For this review, take the finished solid that the model builds, in its own axes (mm). Face numbers are marked on the shaded views. A direction names the side the tool comes from. Round coordinates to 2 decimals unless told otherwise and drop trailing zeros. Write each loop counter-clockwise with the first axis right and the second up, starting at its lowest first coordinate (ties: lowest second). Pieces come first, ordered by that corner, then holes. Notation, with made-up numbers: M 50.25,31.25 L 74.25,31.25 A26 ccw 74.25,61.25 Z; hole C -21,-32 d7. An arc over 180 degrees is marked long. Answer in a Markdown table with one row per item.
```python
from build123d import *

# Parameters (mm, degrees)
F0_W     = 177.8
F0_H     = 33.6000117971
F1_DEPTH = 101.6
F2_R     = 25.4
F3_DEPTH = 33.6010117971
F4_W     = 25.4
F4_H     = 21.9941446124
F5_DEPTH = 101.601


with BuildPart() as f1:
    # F0 (on Front) → F1 (new body)
    with BuildSketch(Plane.XZ):
        with Locations((88.9, 16.8000058986)):
            Rectangle(F0_W, F0_H)
    extrude(amount=F1_DEPTH)

    # F2 (on face) → F3 (cut, through all)
    with BuildSketch(Plane.XY.offset(33.6000117971)):
        with Locations((85.2616652846, -48.5184304416)):
            Circle(F2_R)
    extrude(amount=-F3_DEPTH, mode=Mode.SUBTRACT)

    # F4 (on face) → F5 (cut, through all)
    with BuildSketch(Plane.XZ.offset(101.6)):
        Polygon((177.8, 11.6058671847), (177.8, 33.6000117971), (159.5585218906, 33.6000117971), (152.4, 33.6000117971), (152.4, 11.6058671847), align=None)
        with Locations((12.7, 22.6029394909)):
            Rectangle(F4_W, F4_H)
    extrude(amount=-F5_DEPTH, mode=Mode.SUBTRACT)


solid = f1.part
```
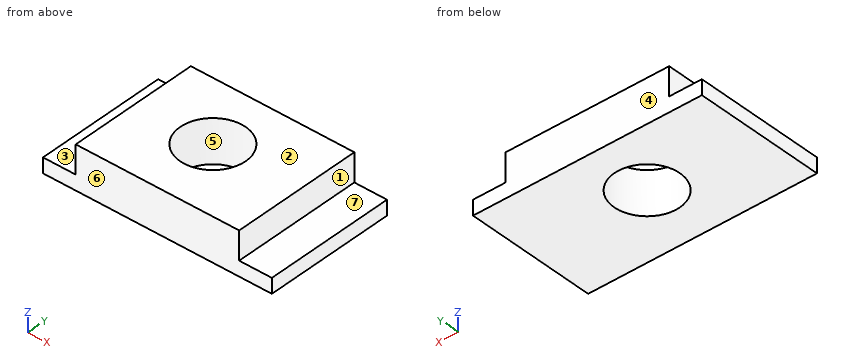
Q1. Mouldability with a two-part tool opening along Y and no side actions: class the marked faces 4, 5, 6 and 7 as +Y half, -Y half, draft (parallel to the pull), parting line (faces both ways), or undercut.
Found:
| item | result |
|---|---|
| face 4 | +Y half |
| face 5 | undercut |
| face 6 | -Y half |
| face 7 | draft |
Q2. Take a section at A-A (y = -67.5). State the section outline as (x, z) points.
Found:
| item | result |
|---|---|
| outline | M 0,0 L 68.38,0 L 68.38,33.6 L 25.4,33.6 L 25.4,11.61 L 0,11.61 Z; M 102.14,0 L 177.8,0 L 177.8,11.61 L 152.4,11.61 L 152.4,33.6 L 102.14,33.6 Z |
Q3. Machinability: for the marked faces 1, 2 and 3, which of the approach directions +Z, -Z, +X, -X, +Y, -Y give a long, thin tool a straight path to every point of the face, cutting with its end or side? Answer none if there is none.
Found:
| item | result |
|---|---|
| face 1 | +Z, +X, +Y, -Y |
| face 2 | +Z, +X, -X, +Y, -Y |
| face 3 | +Z, -X, +Y, -Y |
Q4. Insertion check: P1, Ø3, axis at y = -73.5, z = 26.5, coming from the +X side; P2, Ø6.5, axis at y = -65.5, z = 25, coming from the -X side; P3, Ø12.5, axis at x = 163, y = -70.5, coming from the +Z side. Each pin has a flat end and moves straight along its axis. Give the tip position at first contact, or say it passes through.
Found:
| item | result |
|---|---|
| P1 | x = 152.4 |
| P2 | x = 25.4 |
| P3 | z = 11.61 |
Q5. Take a section at D-D (x = 158). State the section outline as (y, z) points, then the cut area to 3 significant figures.
Found:
| item | result |
|---|---|
| outline | M -101.6,0 L 0,0 L 0,11.61 L -101.6,11.61 Z |
| area | 1,180 mm² |
Q6. Take a section at C-C (x = 105.5). State the section outline as (y, z) points.
Found:
| item | result |
|---|---|
| outline | M -101.6,0 L -63.87,0 L -63.87,33.6 L -101.6,33.6 Z; M -33.17,0 L 0,0 L 0,33.6 L -33.17,33.6 Z |
Q7. For probe 1 along X at (y, z) = (-95.5, 21.5); probe 2 along X at (y, z) = (-30.5, 22.5); probe 3 along Z at (x, y) = (158, -67.5), list the stretches that pass through material, from the lowest coordinate up.
Found:
| item | result |
|---|---|
| probe 1 | 25.4 to 152.4 |
| probe 2 | 25.4 to 67.36, 103.16 to 152.4 |
| probe 3 | 0 to 11.61 |
Q8. Take a section at B-B (y = -92.5). State the section outline as (x, z) points, then the cut area to 3 significant figures.
Found:
| item | result |
|---|---|
| outline | M 0,0 L 177.8,0 L 177.8,11.61 L 152.4,11.61 L 152.4,33.6 L 25.4,33.6 L 25.4,11.61 L 0,11.61 Z |
| area | 4,860 mm² |
